```python
from build123d import *

# Parameters (mm, degrees)
BOSS_EXTRUDE1_DEPTH = 1.5
SKETCH2_R           = 1.1
CUT_EXTRUDE1_DEPTH  = 2.5
FILLET1_R           = 2
SKETCH3_R           = 4
BOSS_EXTRUDE2_DEPTH = 9.5
SKETCH4_R           = 9
BOSS_EXTRUDE3_DEPTH = 9
FILLET2_R           = 1
SKETCH5_R           = 3
BOSS_EXTRUDE4_DEPTH = 3
SKETCH6_R           = 1
BOSS_EXTRUDE5_DEPTH = 10
SKETCH7_R           = 2
CUT_EXTRUDE2_DEPTH  = 1
SKETCH8_R           = 8
CUT_EXTRUDE3_DEPTH  = 1


with BuildPart() as part:
    # Sketch1 → Boss-Extrude1 (new body)
    with BuildSketch(Plane(origin=(0, 0, 0), x_dir=(1, 0, 0), z_dir=(0, 1, 0))):
        with BuildLine():
            Line((-3, 10.062305899), (-3, 3))
            Line((-3, 3), (-10.062305899, 3))
            ThreePointArc((-10.062305899, 3), (-10.5, 0), (-10.062305899, -3))
            Line((-10.062305899, -3), (-3, -3))
            Line((-3, -3), (-3, -10.062305899))
            ThreePointArc((-3, -10.062305899), (0, -10.5), (3, -10.062305899))
            Line((3, -10.062305899), (3, -3))
            Line((3, -3), (10.062305899, -3))
            ThreePointArc((10.062305899, -3), (10.5, 0), (10.062305899, 3))
            Line((10.062305899, 3), (3, 3))
            Line((3, 3), (3, 10.062305899))
            ThreePointArc((3, 10.062305899), (0, 10.5), (-3, 10.062305899))
        make_face()
    extrude(amount=BOSS_EXTRUDE1_DEPTH)

    # Sketch2 → Cut-Extrude1 (cut, through all)
    with BuildSketch(Plane(origin=(0, 1.5, 0), x_dir=(1, 0, 0), z_dir=(0, 1, 0))):
        with Locations((-7.75, 0)):
            Circle(SKETCH2_R)
        with Locations((0, 7.75)):
            Circle(SKETCH2_R)
        with Locations((7.75, 0)):
            Circle(SKETCH2_R)
        with Locations((0, -7.75)):
            Circle(SKETCH2_R)
    extrude(amount=-CUT_EXTRUDE1_DEPTH, mode=Mode.SUBTRACT)

    # Fillet1
    fillet1_edges = [part.edges().sort_by_distance(p)[0] for p in [
        (3, 0.75, 3),
        (3, 0.75, 10.062305899),
        (-3, 0.75, 10.062305899),
        (-3, 0.75, 3),
        (-10.062305899, 0.75, 3),
        (-10.062305899, 0.75, -3),
        (-3, 0.75, -3),
        (-3, 0.75, -10.062305899),
        (3, 0.75, -10.062305899),
        (3, 0.75, -3),
        (10.062305899, 0.75, -3),
        (10.062305899, 0.75, 3),
    ]]
    fillet(fillet1_edges, radius=FILLET1_R)

    # Sketch3 → Boss-Extrude2 (add)
    with BuildSketch(Plane(origin=(0, 1.5, 0), x_dir=(1, 0, 0), z_dir=(0, 1, 0))):
        Circle(SKETCH3_R)
    extrude(amount=BOSS_EXTRUDE2_DEPTH)

    # Sketch4 → Boss-Extrude3 (add)
    with BuildSketch(Plane(origin=(0, 11, 0), x_dir=(1, 0, 0), z_dir=(0, 1, 0))):
        Circle(SKETCH4_R)
    extrude(amount=BOSS_EXTRUDE3_DEPTH)

    # Fillet2
    fillet2_edges = [part.edges().sort_by_distance(p)[0] for p in [
        (-9, 20, 0),
    ]]
    fillet(fillet2_edges, radius=FILLET2_R)

    # Sketch5 → Boss-Extrude4 (add)
    with BuildSketch(Plane(origin=(0, 20, 0), x_dir=(1, 0, 0), z_dir=(0, 1, 0))):
        Circle(SKETCH5_R)
    extrude(amount=BOSS_EXTRUDE4_DEPTH)

    # Sketch6 → Boss-Extrude5 (add)
    with BuildSketch(Plane(origin=(0, 23, 0), x_dir=(1, 0, 0), z_dir=(0, 1, 0))):
        Circle(SKETCH6_R)
    extrude(amount=BOSS_EXTRUDE5_DEPTH)

    # Sketch7 → Cut-Extrude2 (cut)
    with BuildSketch(Plane(origin=(0, 20, 0), x_dir=(1, 0, 0), z_dir=(0, 1, 0))):
        with Locations((-5.5, 0)):
            Circle(SKETCH7_R)
        with Locations((-2.75, 4.763139721)):
            Circle(SKETCH7_R)
        with Locations((2.75, 4.763139721)):
            Circle(SKETCH7_R)
        with Locations((5.5, 0)):
            Circle(SKETCH7_R)
        with Locations((2.75, -4.763139721)):
            Circle(SKETCH7_R)
        with Locations((-2.75, -4.763139721)):
            Circle(SKETCH7_R)
    extrude(amount=-CUT_EXTRUDE2_DEPTH, mode=Mode.SUBTRACT)

    # Sketch8 → Cut-Extrude3 (cut)
    with BuildSketch(Plane(origin=(0, 19, 0), x_dir=(1, 0, 0), z_dir=(0, 1, 0))):
        Circle(SKETCH8_R)
    extrude(amount=-CUT_EXTRUDE3_DEPTH, mode=Mode.SUBTRACT)


solid = part.part
```
Build history of the part. All positions in model axes, mm. A direction names the side the tool comes from. Round coordinates to 2 decimals unless told otherwise and drop trailing zeros. Write each loop counter-clockwise with the first axis right and the second up, starting at its lowest first coordinate (ties: lowest second). Pieces come first, ordered by that corner, then holes. Notation, with made-up numbers: (1, -23.75) -> (6, -23.75) arc R11 cw to (6, -8.75) -> close; hole circle Ø3 at (6, -0.5). An arc over 180 degrees is marked (long way). Put each result on its own line as item: value.
Item 1: Flat gauge pins, fed straight in: P1, Ø10, axis at x = 4, z = -5.5, coming from the +Y side; P2, Ø1.2, axis at y = 0.5, z = -6, coming from the +X side; P3, Ø1.8, axis at x = 0, z = 7.75, coming from the +Y side. Where does each tip first touch, or does it go through?
Here are the results:
P1: stops at y = 23
P2: stops at x = 3
P3: stops at y = 20
Item 2: Slice it at C-C, the plane y = 7.5. Give the cut face in (x, z), plus the area to 3 significant figures.
Here are the results:
outline: circle Ø8 at (0, 0)
area: 50.3 mm^2
Item 3: Slice it at A-A, the plane x = 0. Count the separate pieces of the cut face and the enclosed holes in it, plus the area to 3 significant figures.
Here are the results:
separate pieces: 3
enclosed holes: 1
area: 284 mm^2
Item 4: Tool access for faces 4 (the face through (7, 1, 3)), 5 (the face through (-7, 1, 3)), 6 (the face through (8.766, 0.76, 0.421)), 7 (the face through (-7, 1, -3)), 8 (the face through (0, 28, 1)): list every direction of +Z, -Z, +X, -X, +Y, -Y with a clear straight run to the whole face (end or side of a thin tool).
Here are the results:
face 4: +Z, +X, -Y
face 5: +Z, -X, -Y
face 6: -Y
face 7: -Z, -X, -Y
face 8: +Y
Item 5: Two-plate mould, pull along X, no slides. Class faces 1 (the face through (3, 1, -7)), 2 (the face through (-1.73, 18.51, 7.81)), 3 (the face through (-3, 21, 0)): pulls with the +X half, pulls with the -X half, needs draft (parallel to the pull), parting line crosses it, or undercut.
Here are the results:
face 1: pulls with the +X half
face 2: undercut
face 3: parting line crosses it
Item 6: Slice it at D-D, the plane y = 13. Give the cut face in (x, z), plus the area to 3 significant figures.
Here are the results:
outline: circle Ø18 at (0, 0)
area: 254 mm^2
Item 7: Wall check: probe 1 along Y at (x, z) = (7.5, -0.5); probe 2 along Y at (x, z) = (-7, 2); probe 3 along Y at (x, z) = (0.25, 0.5). Give the ranges that are in metal, low to high. Write a range as from..to.
Here are the results:
probe 1: y = 11..18, 19..20
probe 2: y = 0..1.5, 11..18, 19..20
probe 3: y = 0..18, 19..33
